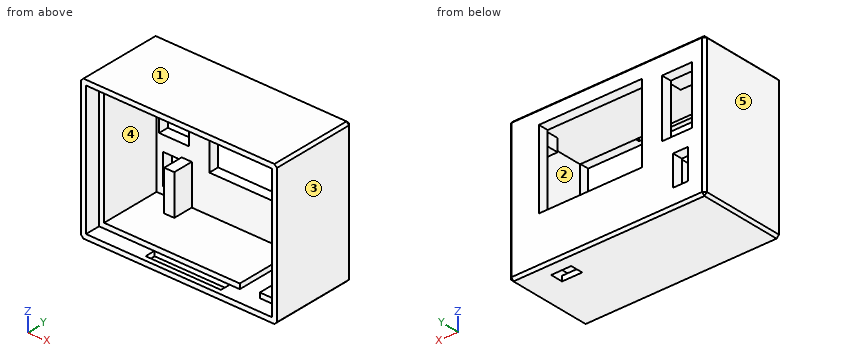
from build123d import *

# Parameters (mm, degrees)
SKETCH_1_W               = 39
SKETCH_1_H               = 28
EXTRUDE_1_DEPTH          = 17
SKETCH_2_W               = 20.5
SKETCH_2_H               = 15.5
CUT_EXTRUDE_1_DEPTH      = 34.228376427
SKETCH_3_W               = 35
SKETCH_3_H               = 24
CUT_EXTRUDE_2_DEPTH      = 15
SKETCH_5_W               = 6
SKETCH_5_H               = 11.5
CUT_EXTRUDE_4_DEPTH      = 34.228376427
SKETCH_7_W               = 3
SKETCH_7_H               = 6
CUT_EXTRUDE_5_DEPTH      = 34.228376427
SKETCH_6_W               = 2.5
SKETCH_6_H               = 8
SKETCH_6_H_2             = 2.5
SKETCH_6_W_2             = 8
SKETCH_6_H_3             = 1.2
SKETCH_6_W_3             = 2
EXTRUDE_2_DEPTH          = 4
SKETCH_8_W               = 37
SKETCH_8_H               = 26
CUT_EXTRUDE_6_DEPTH      = 3
SKETCH_9_W               = 15
SKETCH_9_H               = 2
CUT_EXTRUDE_7_DEPTH      = 0.5
CUT_EXTRUDE_7_DRAFT      = -45
MIRROR_1_COPY_1_SKETCH_W = 15
MIRROR_1_COPY_1_SKETCH_H = 2
MIRROR_1_COPY_1_DEPTH    = 0.5
MIRROR_1_COPY_1_DRAFT    = -45
CUT_EXTRUDE_8_REACH      = 41.882
SKETCH_12_W              = 4
SKETCH_12_H              = 2.5
CHAMFER_1_SIZE           = 0.5
SKETCH_13_W              = 4
SKETCH_13_H              = 1
CUT_EXTRUDE_9_DEPTH      = 11.7


with BuildPart() as part:
    # Эскиз1 → Бобышка-Вытянуть1 (new body)
    with BuildSketch(Plane(origin=(0, 0, 0), x_dir=(1, 0, 0), z_dir=(0, 1, 0))):
        with Locations((-3.25, 3.25)):
            Rectangle(SKETCH_1_W, SKETCH_1_H)
    extrude(amount=EXTRUDE_1_DEPTH)

    # Эскиз2 → Вырез-Вытянуть1 (cut, through all)
    with BuildSketch(Plane(origin=(0, 0, 0), x_dir=(1, 0, 0), z_dir=(0, 1, 0))):
        Rectangle(SKETCH_2_W, SKETCH_2_H)
    extrude(amount=CUT_EXTRUDE_1_DEPTH, mode=Mode.SUBTRACT)

    # Эскиз3 → Вырез-Вытянуть2 (cut)
    with BuildSketch(Plane(origin=(0, 0, 0), x_dir=(1, 0, 0), z_dir=(0, 1, 0))):
        with Locations((-3.25, 3.25)):
            Rectangle(SKETCH_3_W, SKETCH_3_H)
    extrude(amount=CUT_EXTRUDE_2_DEPTH, mode=Mode.SUBTRACT)

    # Эскиз5 → Вырез-Вытянуть4 (cut, through all)
    with BuildSketch(Plane(origin=(0, 0, 0), x_dir=(1, 0, 0), z_dir=(0, 1, 0))):
        with Locations((-17.25, -1)):
            Rectangle(SKETCH_5_W, SKETCH_5_H)
    extrude(amount=CUT_EXTRUDE_4_DEPTH, mode=Mode.SUBTRACT)

    # Эскиз7 → Вырез-Вытянуть5 (cut, through all)
    with BuildSketch(Plane(origin=(0, 0, 0), x_dir=(1, 0, 0), z_dir=(0, 1, 0))):
        with Locations((-17.95, 10.75)):
            Rectangle(SKETCH_7_W, SKETCH_7_H)
    extrude(amount=CUT_EXTRUDE_5_DEPTH, mode=Mode.SUBTRACT)

    # Эскиз6 → Бобышка-Вытянуть2 (add)
    with BuildSketch(Plane.XZ.offset(-15)):
        with Locations((13, -11.25)):
            Rectangle(SKETCH_6_W, SKETCH_6_H)
        with Locations((13, 7.5)):
            Rectangle(SKETCH_6_W, SKETCH_6_H_2)
        with Locations((-16.75, 8.15)):
            Rectangle(SKETCH_6_W_2, SKETCH_6_H_3)
        with Locations((-14.75, -11.25)):
            Rectangle(SKETCH_6_W_3, SKETCH_6_H)
    extrude(amount=EXTRUDE_2_DEPTH)

    # Эскиз8 → Вырез-Вытянуть6 (cut)
    with BuildSketch(Plane(origin=(0, 0, 0), x_dir=(1, 0, 0), z_dir=(0, 1, 0))):
        with Locations((-3.25, 3.25)):
            Rectangle(SKETCH_8_W, SKETCH_8_H)
    extrude(amount=CUT_EXTRUDE_6_DEPTH, mode=Mode.SUBTRACT)


with BuildPart() as cut_extrude_7_tool:
    # Эскиз9 → Вырез-Вытянуть7 (with draft: the straight prism first)
    with BuildSketch(Plane.XY.offset(-16.25)):
        with Locations((-3.25, 2)):
            Rectangle(SKETCH_9_W, SKETCH_9_H)
    extrude(amount=-CUT_EXTRUDE_7_DEPTH)
    # Вырез-Вытянуть7: the draft: its side faces are tilted about the plane it starts from
    cut_extrude_7_sides = [cut_extrude_7_tool.faces().sort_by_distance(p)[0] for p in [
        (-10.75, 2, -16.5),
        (-3.25, 1, -16.5),
        (4.25, 2, -16.5),
        (-3.25, 3, -16.5),
    ]]
    draft(cut_extrude_7_sides, Plane.XY.offset(-16.25), CUT_EXTRUDE_7_DRAFT)


with BuildPart() as part_1:
    add(part.part)

    # Вырез-Вытянуть7: cut by cut_extrude_7_tool
    add(cut_extrude_7_tool.part, mode=Mode.SUBTRACT)


with BuildPart() as mirror_1_copy_1_tool:
    # Зеркальное отражение1 copy 1 sketch → Зеркальное отражение1 copy 1 (with draft: the straight prism first)
    with BuildSketch(Plane(origin=(0, 0, 9.75), x_dir=(1, 0, 0), z_dir=(0, 0, -1))):
        with Locations((-3.25, -2)):
            Rectangle(MIRROR_1_COPY_1_SKETCH_W, MIRROR_1_COPY_1_SKETCH_H)
    extrude(amount=-MIRROR_1_COPY_1_DEPTH)
    # Зеркальное отражение1 copy 1: the draft: its side faces are tilted about the plane it starts from
    mirror_1_copy_1_sides = [mirror_1_copy_1_tool.faces().sort_by_distance(p)[0] for p in [
        (-10.75, 2, 10),
        (-3.25, 1, 10),
        (4.25, 2, 10),
        (-3.25, 3, 10),
    ]]
    draft(mirror_1_copy_1_sides, Plane(origin=(0, 0, 9.75), x_dir=(1, 0, 0), z_dir=(0, 0, -1)), MIRROR_1_COPY_1_DRAFT)


with BuildPart() as part_2:
    add(part_1.part)

    # Зеркальное отражение1 copy 1: cut by mirror_1_copy_1_tool
    add(mirror_1_copy_1_tool.part, mode=Mode.SUBTRACT)

    # Эскиз12 → Вырез-Вытянуть8 (cut, up to next)
    with BuildSketch(Plane(origin=(0, 0, -17.25), x_dir=(-1, 0, 0), z_dir=(0, 0, -1)), mode=Mode.PRIVATE) as cut_extrude_8_sk1:
        with Locations((-8.25, 12.95)):
            Rectangle(SKETCH_12_W, SKETCH_12_H)
    cut_extrude_8_tool1 = extrude(cut_extrude_8_sk1.sketch, amount=-CUT_EXTRUDE_8_REACH, mode=Mode.PRIVATE) & part_2.part
    add(cut_extrude_8_tool1.solids().sort_by_distance((8.25, 12.95, -17.25))[0], mode=Mode.SUBTRACT)

    # Фаска1
    chamfer_1_edges = [part_2.edges().sort_by_distance(p)[0] for p in [
        (16.25, 17, -3.25),
        (-3.25, 17, -17.25),
        (-22.75, 17, -3.25),
        (-22.75, 8.5, -17.25),
        (16.25, 8.5, -17.25),
        (16.25, 8.5, 10.75),
        (-22.75, 8.5, 10.75),
        (-3.25, 17, 10.75),
    ]]
    chamfer(chamfer_1_edges, length=CHAMFER_1_SIZE)

    # Эскиз13 → Вырез-Вытянуть9 (cut)
    with BuildSketch(Plane(origin=(0, 0, 0), x_dir=(1, 0, 0), z_dir=(0, 1, 0))):
        with Locations((8.25, 15.75)):
            Rectangle(SKETCH_13_W, SKETCH_13_H)
    extrude(amount=CUT_EXTRUDE_9_DEPTH, mode=Mode.SUBTRACT)


solid = part_2.part
Can you work these out from the model? Positions are in its coordinate system, mm. Face numbers are marked on the shaded views. A direction names the side the tool comes from. Coordinates: 2 decimals unless noted, no trailing zeros. Loops run counter-clockwise (first coordinate to the right, second up) from the corner with the lowest first, then second, coordinate; pieces in that order, holes last. Notation, with made-up numbers: M 80.5,74 L 84.5,74 A25 cw 84.5,112 Z; hole C 56,40.5 d7. An arc over 180 degrees is marked long. Return JSON: item names as keys, results as strings. Group by question number.
Item 1: Imagine slicing it at C-C (y = 5.75). Please give me the cut outline in (x, z).
Item 2: I'm going to push flat-ended pins straight in: pin 1 Ø1 at (x, z) = (-6, 8) entering from -Y; pin 2 Ø6 at (x, z) = (-14.5, 5.5) entering from -Y. Where does each tip first touch, or does it pass through?
Item 3: If I drill on L1, parallel to X at y = 13.25, z = -12.25; L2, parallel to X at y = 9.25, z = -10.5; L3, parallel to Z at x = -6, y = 8, over which ranges is the centre line in solid material (lowest first)? Write a range as from..to.
Item 4: Imagine slicing it at D-D (x = -4). Please give me the cut outline in (y, z), and give its area (4 significant figures).
Item 5: Imagine slicing it at B-B (z = -12.5). Please give me the cut outline in (x, y), and give its area (3 significant figures).
Item 6: On a 3-axis mill with a long thin cutter (end or side, diameter ignored), from which of +Z, -Z, +X, -X, +Y, -Y can I reach the whole of each face in a straight line? I mean the marked faces 1 and 2. Say none if no direction works.
Item 7: Thinking about a two-plate mould opening in X: for the marked faces 3, 4 and 5, which applies, released by +X, released by -X, zero draft, split by the parting line, or undercut?
Item 8: Imagine slicing it at A-A (x = 7.5). Please give me the cut outline in (y, z).
Verdict:
{
 "1": {"outline": "M -22.75,-16.75 L -22.25,-17.25 L 15.75,-17.25 L 16.25,-16.75 L 16.25,10.25 L 15.75,10.75 L -22.25,10.75 L -22.75,10.25 Z; hole M -20.75,-15.25 L 6.25,-15.25 L 6.25,-16.25 L 10.25,-16.25 L 10.25,-15.25 L 14.25,-15.25 L 14.25,8.75 L -20.75,8.75 Z"},
 "2": {"pin 1": "stops at y = 15", "pin 2": "stops at y = 11"},
 "3": {"L1": "x = -22.75..-20.75, -15.75..-13.75, 11.75..16.25", "L2": "x = -22.75..-20.75, 14.25..16.25", "L3": "z = -17.25..-15.25, 8.75..10.75"},
 "4": {"outline": "M 0,-17.25 L 16.5,-17.25 L 17,-16.75 L 17,-7.75 L 15,-7.75 L 15,-15.25 L 3,-15.25 L 3,-16.25 L 2.5,-16.75 L 1.5,-16.75 L 1,-16.25 L 0,-16.25 Z; M 0,9.75 L 1,9.75 L 1.5,10.25 L 2.5,10.25 L 3,9.75 L 3,8.75 L 15,8.75 L 15,7.75 L 17,7.75 L 17,10.25 L 16.5,10.75 L 0,10.75 Z", "area": "77.25 mm^2"},
 "5": {"outline": "M -22.75,0 L -21.75,0 L -21.75,3 L -20.75,3 L -20.75,15 L -19.45,15 L -19.45,17 L -22.25,17 L -22.75,16.5 Z; M -16.45,15 L -15.75,15 L -15.75,11 L -13.75,11 L -13.75,15 L 11.75,15 L 11.75,11 L 14.25,11 L 14.25,3 L 15.25,3 L 15.25,0 L 16.25,0 L 16.25,16.5 L 15.75,17 L -16.45,17 Z", "area": "144 mm^2"},
 "6": {"face 1": "+Z, +X, -X, +Y, -Y", "face 2": "-Y"},
 "7": {"face 3": "released by +X", "face 4": "undercut", "face 5": "released by -X"},
 "8": {"outline": "M 0,-17.25 L 11.7,-17.25 L 11.7,-16.25 L 0,-16.25 Z; M 0,9.75 L 3,9.75 L 3,8.75 L 15,8.75 L 15,7.75 L 17,7.75 L 17,10.25 L 16.5,10.75 L 0,10.75 Z; M 14.2,-17.25 L 16.5,-17.25 L 17,-16.75 L 17,-7.75 L 15,-7.75 L 15,-15.25 L 14.2,-15.25 Z"}
}
